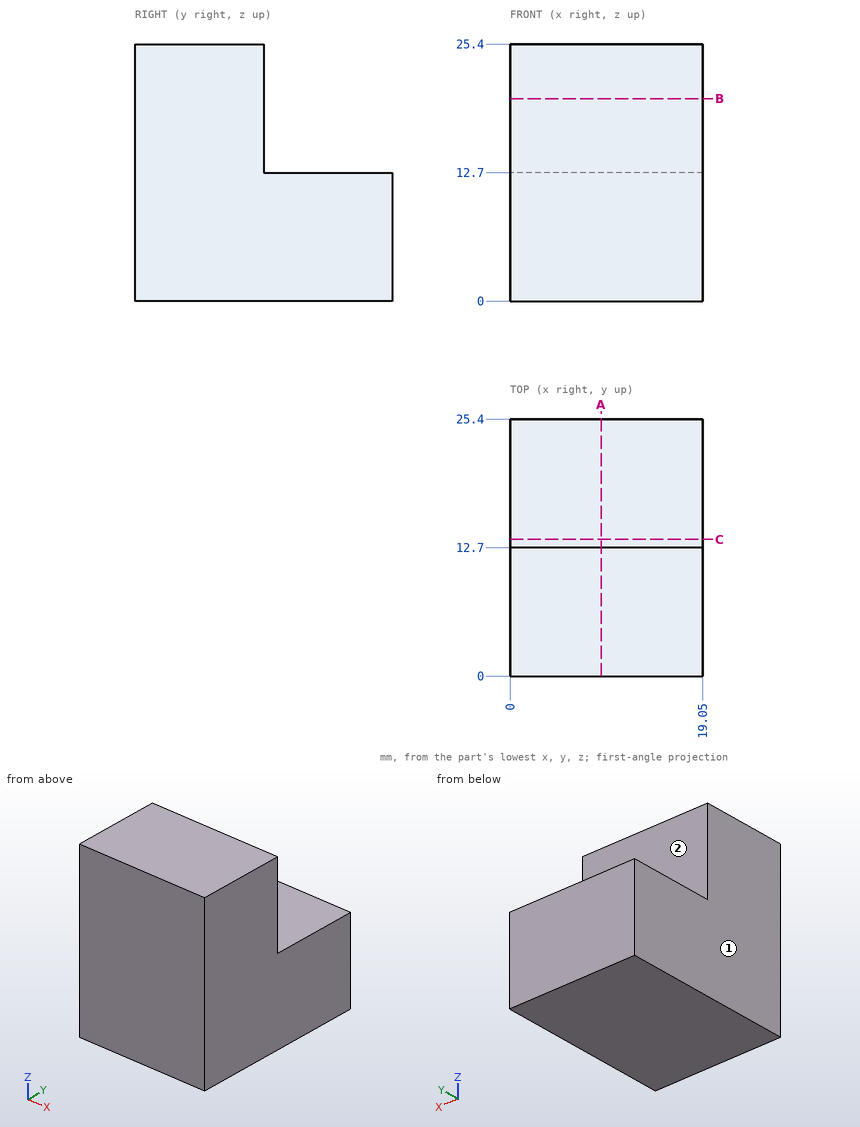
Geometry: see drawing. Coordinates: mm, zero at the bounding-box minimum. A direction names the side the tool comes from. Round coordinates to 2 decimals unless told otherwise and drop trailing zeros. Loops run counter-clockwise (first coordinate to the right, second up) from the corner with the lowest first, then second, coordinate; pieces in that order, holes last. Notation, with made-up numbers: (-9.5, -1.75) - (20.5, -1.75) arc R17 ccw to (20.5, 8.25) - close; hole circle Ø11 at (38, 22.25). An arc over 180 degrees is marked (long way). One line per item, written item: value. Start each with the question number.
(1) Section A-A, the plane x = 9. Return loops of the section in (y, z), plus the area to 3 significant figures.
(2) Contact query for flat-ended pins moving along their axis: P1, Ø4, axis at x = 10.5, y = 17.5, coming from the +Z side; P2, Ø10, axis at y = 3.5, z = 20.5, coming from the -X side; P3, Ø6, axis at x = 4, z = 17, coming from the +Y side. Output: stop coordinate, or through.
(3) Section B-B, the plane z = 20. Return loops of the section in (x, y).
(4) Ray query, line 1 (Y direction, x = 18, z = 14.5). Return the intervals inside material, ascending. Write a range as [from, to].
(5) Access query for the marked faces 1 and 2. Directions: +Z, -Z, +X, -X, +Y, -Y. A direction counts if a zero-diameter tool reaches every point of the face in a straight line with its end or side. Return the directions, or none.
Results below:
1. outline: (0, 0) - (25.4, 0) - (25.4, 12.7) - (12.7, 12.7) - (12.7, 25.4) - (0, 25.4) - close
1. area: 484 mm^2
2. P1: z = 12.7
2. P2: x = 0
2. P3: y = 12.7
3. outline: (0, 0) - (19.05, 0) - (19.05, 12.7) - (0, 12.7) - close
4. line 1: [0, 12.7]
5. face 1: +Z, -Z, -X, +Y, -Y
5. face 2: +Z, +X, -X, +Y
